from build123d import *

# Parameters (mm, degrees)
SKETCH1_W           = 20
SKETCH1_H           = 49.25
BOSS_EXTRUDE1_DEPTH = 0.6
SKETCH2_W           = 23
SKETCH2_H           = 52.25
BOSS_EXTRUDE2_DEPTH = 1
SKETCH3_R           = 3.5
CUT_EXTRUDE1_DEPTH  = 10


with BuildPart() as part:
    # Sketch1 → Boss-Extrude1 (new body)
    with BuildSketch(Plane(origin=(0, 7.5, 0), x_dir=(1, 0, 0), z_dir=(0, 1, 0))):
        with Locations((10, 25.375)):
            Rectangle(SKETCH1_W, SKETCH1_H)
    extrude(amount=-BOSS_EXTRUDE1_DEPTH)

    # Sketch2 → Boss-Extrude2 (add)
    with BuildSketch(Plane(origin=(0, 7.5, 0), x_dir=(1, 0, 0), z_dir=(0, 1, 0))):
        with Locations((10, 25.375)):
            Rectangle(SKETCH2_W, SKETCH2_H)
    extrude(amount=BOSS_EXTRUDE2_DEPTH)

    # Sketch3 → Cut-Extrude1 (cut)
    with BuildSketch(Plane(origin=(0, 8.5, 0), x_dir=(1, 0, 0), z_dir=(0, 1, 0))):
        with Locations((10, 41.5)):
            Circle(SKETCH3_R)
    extrude(amount=-CUT_EXTRUDE1_DEPTH, mode=Mode.SUBTRACT)


solid = part.part
Geometry check sheet. Reference: the model listing, model coordinates, mm. Give positions to 0.01 mm unless a question says otherwise; leave off trailing zeros. Write each loop counter-clockwise with the first axis right and the second up, starting at its lowest first coordinate (ties: lowest second). Pieces come first, ordered by that corner, then holes. Notation, with made-up numbers: M 84.25,-5 L 118.25,-5 A7 ccw 118.25,4 Z; hole C -7.5,-17.5 d9. An arc over 180 degrees is marked long. Answer as CSV lines item,"result". Start each with the question number.
Q1. Section check A-A, the plane z = -41.5. Record the cut outline in (x, y).
Q2. Release check for a two-part mould opening along Z. For faces 1 (the face through (10, 8, -51.5)), 2 (the face through (10, 8, -45)), 3 (the face through (-1.5, 8, -25)), 4 (the face through (10, 8, 0.75)) record: pulls with the +Z half, pulls with the -Z half, needs draft (parallel to the pull), parting line crosses it, or undercut.
Q3. Go/stop test with a flat-tipped pin: pin 1 (0.7 mm diameter, centred on y = 7, z = -31.5, fed in from -X). Record where the tip stops, or that it passes through.
Q4. Material ranges on L1, parallel to Z at x = 10, y = 7.35; L2, parallel to X at y = 7.9, z = -41.5; L3, parallel to Z at x = 10, y = 7.8, recorded low to high.
Q5. Section check B-B, the plane x = 10. Record the cut outline in (y, z).
Q6. Section check D-D, the plane y = 8.1. Record the cut outline in (x, z), then the cut area to 3 significant figures.
Q7. Section check C-C, the plane z = -14.5. Record the cut outline in (x, y).
Geometry says:
1,outline,"M -1.5,7.5 L 0,7.5 L 0,6.9 L 6.5,6.9 L 6.5,8.5 L -1.5,8.5 Z; M 13.5,6.9 L 20,6.9 L 20,7.5 L 21.5,7.5 L 21.5,8.5 L 13.5,8.5 Z"
2,face 1,"pulls with the -Z half"
2,face 2,"undercut"
2,face 3,"needs draft"
2,face 4,"pulls with the +Z half"
3,pin 1,"x = 0"
4,L1,"-50 to -45, -38 to -0.75"
4,L2,"-1.5 to 6.5, 13.5 to 21.5"
4,L3,"-51.5 to -45, -38 to 0.75"
5,outline,"M 6.9,-50 L 7.5,-50 L 7.5,-51.5 L 8.5,-51.5 L 8.5,-45 L 6.9,-45 Z; M 6.9,-38 L 8.5,-38 L 8.5,0.75 L 7.5,0.75 L 7.5,-0.75 L 6.9,-0.75 Z"
6,outline,"M -1.5,-51.5 L 21.5,-51.5 L 21.5,0.75 L -1.5,0.75 Z; hole C 10,-41.5 d7"
6,area,"1,160 mm^2"
7,outline,"M -1.5,7.5 L 0,7.5 L 0,6.9 L 20,6.9 L 20,7.5 L 21.5,7.5 L 21.5,8.5 L -1.5,8.5 Z"
